Geometry check sheet. Reference: the model listing, model coordinates, mm. A direction names the side the tool comes from. Coordinates: 2 decimals unless noted, no trailing zeros. Write each loop counter-clockwise with the first axis right and the second up, starting at its lowest first coordinate (ties: lowest second). Pieces come first, ordered by that corner, then holes. Notation, with made-up numbers: (30, 58.5) -> (86, 58.5) arc R8 ccw to (86, 72.5) -> close; hole circle Ø6 at (53.5, 5.5). An arc over 180 degrees is marked (long way). One line per question, with ' | ' between items.
```python
from build123d import *


with BuildPart() as part:
    # Skizze1 → Rotation1 (revolve)
    with BuildSketch(Plane.XY, mode=Mode.PRIVATE) as rotation1_sk:
        Polygon((4, 0), (8, 0), (8, -3.7), (6, -3.7), (6, -9.7), (8, -9.7), (8, -12.7), (4.5, -12.7), (4.5, -14.2), (8, -14.2), (8, -15.2), (4.5, -15.2), (4.5, -16.7), (11, -16.7), (11, -17.7), (3.5, -17.7), (3.5, -19.7), (10.55, -19.7), (10.55, -20.7), (3.05, -20.7), (3.05, -23.7), (10.55, -23.7), (10.55, -24.7), (3.5, -24.7), (3.5, -26.7), (11, -26.7), (11, -27.7), (7, -27.7), (7, -29.2), (11, -29.2), (11, -30.2), (3.5, -30.2), (3.5, -32.2), (10.55, -32.2), (10.55, -33.2), (3.05, -33.2), (3.05, -35.45), (10.55, -35.45), (10.55, -36.45), (3.05, -36.45), (3.05, -38.7), (10.55, -38.7), (10.55, -39.7), (3.65, -39.7), (3.65, -41.7), (11.15, -41.7), (11.15, -42.7), (2.75, -42.7), (2.75, -44.8), (3, -44.8), (3, -49.8), (2, -49.8), (2, -7.900415076), (4, -6.5), align=None)
    revolve(rotation1_sk.sketch.rotate(Axis((0, 0, 0), (0, 1, 0)), 90), axis=Axis((0, 0, 0), (0, 1, 0)))


solid = part.part
```
(1) Depth check by flat-ended pin: P1, Ø3, axis at y = -33, z = -5.5, coming from the -X side; P2, Ø3, axis at x = 6, z = -8.5, coming from the +Y side; P3, Ø3, axis at x = 4.5, z = 1.5, coming from the -Y side; P4, Ø2, axis at y = -8, z = -8.5, coming from the +X side. Enter the tip coordinate at first touch or a pass-through.
Answers below:
P1: stops at x = -9.76 | P2: stops at y = -16.7 | P3: stops at y = -42.7 | P4: passes through
(2) Material ranges on line 1 (X direction, y = -4, z = 0); line 2 (Y direction, x = 9.5, z = 4.75); line 3 (X direction, y = -19, z = 0), recorded low to high.
Answers below:
line 1: x = -6 to -4, 4 to 6 | line 2: y = -42.7 to -41.7, -30.2 to -29.2, -27.7 to -26.7, -17.7 to -16.7 | line 3: x = -3.5 to -2, 2 to 3.5
(3) Cross-section at A-A (y = -16). Record the cut outline in (x, z), plus the area to 3 significant figures.
Answers below:
outline: circle Ø9 at (0, 0); hole circle Ø4 at (0, 0) | area: 51.1 mm²
(4) Cross-section at B-B (x = 9.5). Count the separate pieces of the cut face and the enclosed holes in it, plus the area to 3 significant figures.
Answers below:
separate pieces: 9 | enclosed holes: 0 | area: 90.8 mm²
(5) Tool access check on faces 4 (the face through (2, -29, 0)), 5 (the face through (0, -24.7, -5)). Record the directions out of +Z, -Z, +X, -X, +Y, -Y that give a thin tool (end or side, any length) a straight path to the whole face; none if there is none.
Answers below:
face 4: +Y, -Y | face 5: none
(6) Draft check along Y on faces 1 (the face through (10.74, -27.21, 2.38)), 2 (the face through (3.105, -31.214, -1.615)), 3 (the face through (-3.169, -39.207, -10.063)). Enter one of: pulls with the +Y half, pulls with the -Y half, needs draft (parallel to the pull), parting line crosses it, or undercut.
Answers below:
face 1: needs draft | face 2: undercut | face 3: undercut
